Autodesk Inventor part; units mm, degrees
ref_plane "Start Plane" through (0, 0, 25.4) normal (0, 0, 1) x (1, 0, 0)
ref_plane "End Plane" through (0, 0, 482.6) normal (0, 0, 1) x (1, 0, 0)
ref_plane "YZ Plane" through (0, 0, 0) normal (1, 0, 0) x (0, 1, 0)
ref_plane "Start Plane" through (0, 0, 25.4) normal (0, 0, 1) x (1, 0, 0)
ref_plane "End Plane" through (0, 0, 482.6) normal (0, 0, 1) x (1, 0, 0)
sketch "Sketch" plane through (0, 0, 0) normal (0, 0, 1) x (1, 0, 0)
  line L0 (-25.4, -19.05) -> (-25.4, 19.05)
  line L1 (-19.05, 25.4) -> (19.05, 25.4)
  line L2 (25.4, 19.05) -> (25.4, -19.05)
  line L3 (19.05, -25.4) -> (-19.05, -25.4)
  arc A0 (-25.4, -19.05) -> (-19.05, -25.4) centre (-19.05, -19.05) ccw
  arc A1 (-19.05, 25.4) -> (-25.4, 19.05) centre (-19.05, 19.05) ccw
  arc A2 (25.4, 19.05) -> (19.05, 25.4) centre (19.05, 19.05) ccw
  arc A3 (19.05, -25.4) -> (25.4, -19.05) centre (19.05, -19.05) ccw
  arc A4 (-19.05, 22.225) -> (-22.225, 19.05) centre (-19.05, 19.05) ccw
  line L4 (-19.05, 22.225) -> (19.05, 22.225)
  arc A5 (22.225, 19.05) -> (19.05, 22.225) centre (19.05, 19.05) ccw
  line L5 (22.225, 19.05) -> (22.225, -19.05)
  arc A6 (19.05, -22.225) -> (22.225, -19.05) centre (19.05, -19.05) ccw
  line L6 (19.05, -22.225) -> (-19.05, -22.225)
  arc A7 (-22.225, -19.05) -> (-19.05, -22.225) centre (-19.05, -19.05) ccw
  line L7 (-22.225, -19.05) -> (-22.225, 19.05)
  line L8 (0, 37.4012) -> (0, -37.4012) construction
  line L9 (-37.4012, 0) -> (37.4012, 0) construction
  dimension "d10" = 50.8
  dimension "d11" = 50.8
  dimension "d12" = 3.175
  dimension "d15" = 25.4
  dimension "d16" = 25.4
  dimension "d17" = 6.35
extrude "Body" add sketch "Sketch" along normal up to surface (457.2 mm away) from surface at 25.4
sketch "Sketch3" plane through (0, 0, 0) normal (0, 0, 1) x (1, 0, 0)
  line L0 (0, 0) -> (10, 0)
ref_plane "Work Plane3" through (0, 0, 0) normal (0, -1, 0) x (1, 0, 0)
sketch "Sketch4" plane through (0, 0, 0) normal (0, -1, 0) x (1, 0, 0)
  line L0 (-2, 25.4) -> (12, 25.4)
  line L1 (-2, 482.6) -> (12, 482.6)
  dimension "d19" = 457.2
equation "\"d10\" = G_H"
equation "\"d11\" = G_W"
equation "\"d12\" = G_T"
equation "\"d15\" = 0.5 * d10"
equation "\"d16\" = 0.5 * d11"
equation "\"d17\" = G_IR"
equation "\"d3\" = G_L"
equation "\"G_W\" = 50.8"
equation "\"G_H\" = 50.8"
equation "\"G_T\" = 3.175"
equation "\"G_IR\" = 6.35"
equation "\"G_L\" = d19"
equation "\"G_OFFSET_START\" = -25.4"
equation "\"G_OFFSET_END\" = -25.4"
equation "\"d13\" = -G_OFFSET_START"
equation "\"d14\" = G_OFFSET_END + B_L"
equation "\"B_L\" = 508"
properties part number "AISC - 2 x 2 x 1/8 - 18" material "Steel, Mild"
Input: part model. Units: mm. Frame: model coordinates. A direction names the side the tool comes from. Round coordinates to 2 decimals unless told otherwise and drop trailing zeros. Loops run counter-clockwise (first coordinate to the right, second up) from the corner with the lowest first, then second, coordinate; pieces in that order, holes last. Notation, with made-up numbers: (85, 80.25) -> (115, 80.25) arc R20 ccw to (115, 92.25) -> close; hole circle Ø9 at (16.5, 20.5). An arc over 180 degrees is marked (long way). Write each question's results on one line, items separated by ' | '.
1. Set-up query: faces 1 (the face through (0, -22.225, 251)), 2 (the face through (-0.1, -22.5, 25.4)). Return all of +Z, -Z, +X, -X, +Y, -Y with unobstructed straight access to the full face (end or side cutting, diameter ignored); none if empty.
Geometry results:
face 1: +Z, -Z | face 2: -Z, +X, -X, +Y, -Y
2. Section C-C (z = 203). Return loops of the section in (x, y) (3 decimals), and give its area (3 significant figures).
Geometry results:
outline: (-25.4, -19.05) arc R6.35 ccw to (-19.05, -25.4) -> (19.05, -25.4) arc R6.35 ccw to (25.4, -19.05) -> (25.4, 19.05) arc R6.35 ccw to (19.05, 25.4) -> (-19.05, 25.4) arc R6.35 ccw to (-25.4, 19.05) -> close; hole (-22.225, -19.05) arc R3.175 ccw to (-19.05, -22.225) -> (19.05, -22.225) arc R3.175 ccw to (22.225, -19.05) -> (22.225, 19.05) arc R3.175 ccw to (19.05, 22.225) -> (-19.05, 22.225) arc R3.175 ccw to (-22.225, 19.05) -> close | area: 579 mm2
3. Ray query, line 1 (Y direction, x = -10.5, z = 55.5) (3 decimals); line 2 (X direction, y = -21, z = 249). Return the intervals inside material, ascending. Write a range as from..to.
Geometry results:
line 1: -25.4..-22.225, 22.225..25.4 | line 2: -25.09..-21.56, 21.56..25.09
4. Mould query, pull axis Y, two halves, no side actions, for faces 3 (the face through (0, -25.4, 251)), 4 (the face through (25.4, 0, 251)), 5 (the face through (0, 22.225, 251)). Classes: +Y half, -Y half, draft (parallel to the pull), parting line (faces both ways), or undercut.
Geometry results:
face 3: -Y half | face 4: draft | face 5: undercut
5. Section A-A (x = 8). Return loops of the section in (y, z) (3 decimals).
Geometry results:
outline: (-25.4, 25.4) -> (-22.225, 25.4) -> (-22.225, 482.6) -> (-25.4, 482.6) -> close; (22.225, 25.4) -> (25.4, 25.4) -> (25.4, 482.6) -> (22.225, 482.6) -> close
